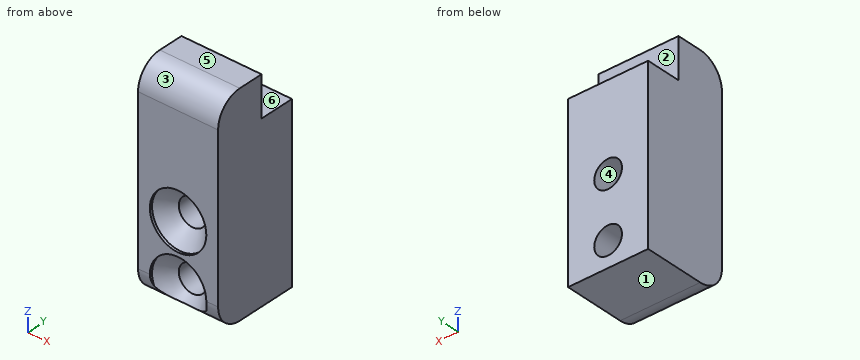
```python
from build123d import *

# Parameters (mm, degrees)
RESSALTO_EXTRUS_O1_DEPTH            = 7.94
FILETE1_R                           = 5
ESCAREADO_PARA_SFHCS_M51_AT_2_COUNT = 2
ESCAREADO_PARA_SFHCS_M51_AT_2_PITCH = 12
ESCAREADO_PARA_SFHCS_M51_AT_3_COUNT = 2
ESCAREADO_PARA_SFHCS_M51_AT_3_PITCH = 67.209946437
ESCAREADO_PARA_SFHCS_M51_AT_4_COUNT = 2
ESCAREADO_PARA_SFHCS_M51_AT_4_PITCH = 66.13


with BuildPart() as part:
    # Esboço1 → Ressalto-extrusão1 (new, symmetric)
    with BuildSketch(Plane(origin=(0, 0, 0), x_dir=(0, 0, -1), z_dir=(1, 0, 0))):
        Polygon((-17, -8.5), (17, -8.5), (17, 8.5), (-17, 8.5), (-17, 1.5), (-25, 1.5), (-25, -8.5), align=None)
    extrude(amount=RESSALTO_EXTRUS_O1_DEPTH, both=True)

    # Filete1
    filete1_edges = [part.edges().sort_by_distance(p)[0] for p in [
        (0, -8.5, -17),
        (0, -8.5, 25),
    ]]
    fillet(filete1_edges, radius=FILETE1_R)

    # Esboço3 → Escareado para SFHCS M51 (revolve, cut)
    with BuildSketch(Plane(origin=(0, -8.5, -12), x_dir=(0, 0, -1), z_dir=(1, 0, 0))):
        Polygon((0, 0), (0, 31.652366702), (2.75, 30), (2.75, 3.35), (5.6, 0.5), (5.6, 0), align=None)
    escareado_para_sfhcs_m51 = revolve(axis=Axis((0, -14.85, -12), (0, 1, 0)), mode=Mode.SUBTRACT)

    # Escareado para SFHCS M51 at 2: Escareado para SFHCS M51 ×2
    with Locations(*[(0, 0, i * ESCAREADO_PARA_SFHCS_M51_AT_2_PITCH) for i in range(1, ESCAREADO_PARA_SFHCS_M51_AT_2_COUNT)]):
        add(escareado_para_sfhcs_m51, mode=Mode.SUBTRACT)

    # Escareado para SFHCS M51 at 3: Escareado para SFHCS M51 ×2
    with Locations(*[Vector(-0.9839317468056482, 0, 0.17854500168861018) * (i * ESCAREADO_PARA_SFHCS_M51_AT_3_PITCH) for i in range(1, ESCAREADO_PARA_SFHCS_M51_AT_3_COUNT)]):
        add(escareado_para_sfhcs_m51, mode=Mode.SUBTRACT)

    # Escareado para SFHCS M51 at 4: Escareado para SFHCS M51 ×2
    with Locations(*[(-i * ESCAREADO_PARA_SFHCS_M51_AT_4_PITCH, 0, 0) for i in range(1, ESCAREADO_PARA_SFHCS_M51_AT_4_COUNT)]):
        add(escareado_para_sfhcs_m51, mode=Mode.SUBTRACT)


solid = part.part
```
The model under review builds one solid part; all positions refer to its coordinate system, in mm. Face numbers are marked on the shaded views. A direction names the side the tool comes from. Round coordinates to 2 decimals unless told otherwise and drop trailing zeros. Order: outer loops, then holes, each group sorted by start corner. A loop starts at its lowest first (then second) coordinate and runs counter-clockwise, first axis right, second up. Notation, with made-up numbers: M 8,-20.5 L 37,-20.5 A33 cw 37,11.5 Z; hole C 66,41 d6. An arc over 180 degrees is marked long. Use a Markdown table: item, result.
1) Consider section C-C (x = 6.25). Write out the cut boundary in (y, z).
Report:
| item | result |
|---|---|
| outline | M -8.5,-12 A5 ccw -3.5,-17 L 8.5,-17 L 8.5,17 L 1.5,17 L 1.5,25 L -3.5,25 A5 ccw -8.5,20 Z |
2) Consider section A-A (z = 0). Write out the cut boundary in (x, y), then the cut area to 3 significant figures.
Report:
| item | result |
|---|---|
| outline | M -7.94,-8.5 L -5.6,-8.5 L -5.6,-8 L -2.75,-5.15 L -2.75,8.5 L -7.94,8.5 Z; M 2.75,-5.15 L 5.6,-8 L 5.6,-8.5 L 7.94,-8.5 L 7.94,8.5 L 2.75,8.5 Z |
| area | 165 mm^2 |
3) Consider section D-D (x = 0). Write out the cut boundary in (y, z).
Report:
| item | result |
|---|---|
| outline | M -8.5,-6.4 L -8,-6.4 L -5.15,-9.25 L 8.5,-9.25 L 8.5,-2.75 L -5.15,-2.75 L -8,-5.6 L -8.5,-5.6 Z; M -8.5,5.6 L -8,5.6 L -5.15,2.75 L 8.5,2.75 L 8.5,17 L 1.5,17 L 1.5,25 L -3.5,25 A5 ccw -8.5,20 Z; M -6.44,-16.04 A5 ccw -3.5,-17 L 8.5,-17 L 8.5,-14.75 L -5.15,-14.75 Z |
4) Tool access review of the marked faces 5 and 6: name each direction out of +Z, -Z, +X, -X, +Y, -Y from which nothing blocks a thin tool from reaching the whole face with its end or side.
Report:
| item | result |
|---|---|
| face 5 | +Z, +X, -X, +Y, -Y |
| face 6 | +Z, +X, -X, +Y |
5) Consider section B-B (y = 5.5). Write out the cut boundary in (x, z), then the cut area to 3 significant figures.
Report:
| item | result |
|---|---|
| outline | M -7.94,-17 L 7.94,-17 L 7.94,17 L -7.94,17 Z; hole C 0,-12 d5.5; hole C 0,0 d5.5 |
| area | 492 mm^2 |
6) Insertion check: pin 1 (1 mm diameter, centred on x = -3, z = 2.5, fed in from -Y); pin 2 (2.5 mm diameter, centred on x = -3.5, z = 21, fed in from +Y); pin 3 (5 mm diameter, centred on x = 0, z = -12, fed in from -Y); pin 4 (5.5 mm diameter, centred on x = 1, y = 5.5, fed in from +Z). Each pin has a flat end and moves straight along its axis. Give the tip position at first contact, or say it passes through.
Report:
| item | result |
|---|---|
| pin 1 | y = -6.81 |
| pin 2 | y = 1.5 |
| pin 3 | through |
| pin 4 | z = 17 |
7) Draft analysis for pull direction Z (two halves, no side actions). For the marked faces 1, 2, 3 and 4, state which applies: released by +Z, released by -Z, zero draft, split by the parting line, or undercut.
Report:
| item | result |
|---|---|
| face 1 | released by -Z |
| face 2 | zero draft |
| face 3 | released by +Z |
| face 4 | undercut |
8) Wall thickness on line 1 along Z through (x, y) = (0, 3.5); line 2 along X through (y, z) = (4.5, 0); line 3 along Z through (x, y) = (-0.5, -2.25): over which ranges is each line inside the solid? List them lowest first. Write a range as [from, to].
Report:
| item | result |
|---|---|
| line 1 | [-17, -14.75], [-9.25, -2.75], [2.75, 17] |
| line 2 | [-7.94, -2.75], [2.75, 7.94] |
| line 3 | [-17, -14.7], [-9.3, -2.7], [2.7, 25] |
